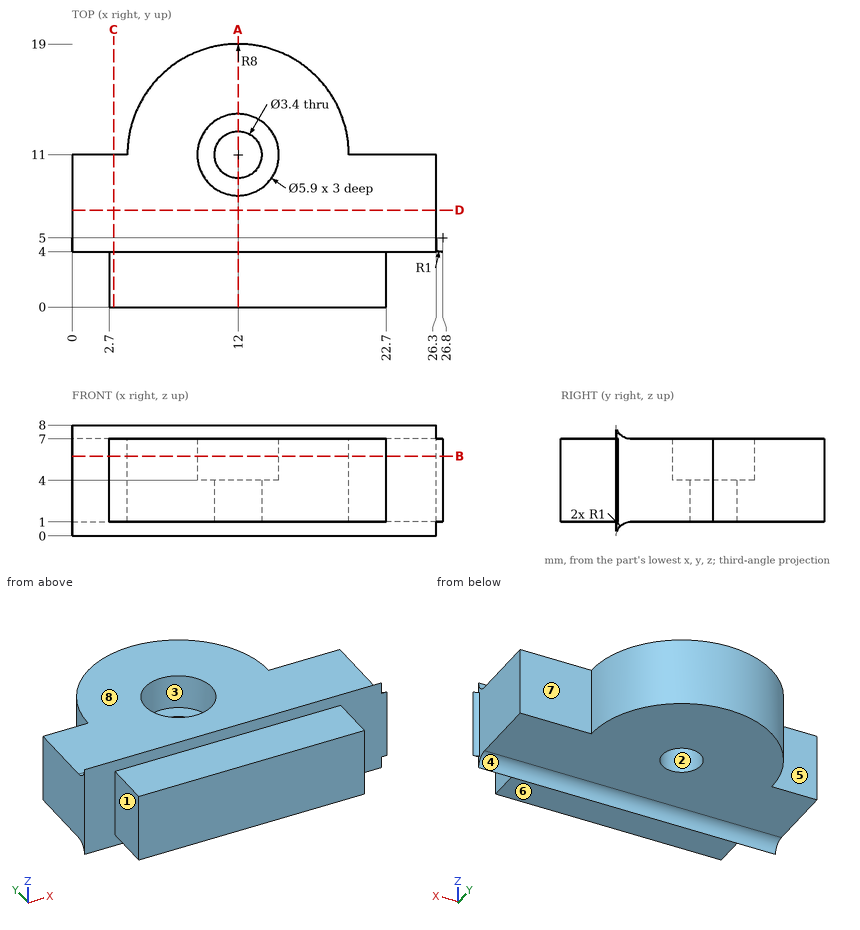
The drawing under review shows one solid part. Ordinate dimensions are in mm from its lowest x, y, z. A direction names the side the tool comes from. Round coordinates to 2 decimals unless told otherwise and drop trailing zeros. Write each loop counter-clockwise with the first axis right and the second up, starting at its lowest first coordinate (ties: lowest second). Pieces come first, ordered by that corner, then holes. Notation, with made-up numbers: (41, 22.25) - (58, 22.25) arc R22 ccw to (58, 35.25) - close; hole circle Ø6 at (54.25, 83). An arc over 180 degrees is marked (long way). Use one line per item in the form item = value.
Q1. Insertion check: pin 1 Ø1.5 at (x, y) = (12.5, 4) entering from -Z; pin 2 Ø2 at (y, z) = (10, 3) entering from +X; pin 3 Ø2 at (x, y) = (14, 2.5) entering from -Z; pin 4 Ø2 at (x, z) = (6, 5.5) entering from -Y. Each pin has a flat end and moves straight along its axis. Give the tip position at first contact, or say it passes through.
Answer key:
pin_1 = 0
pin_2 = 26.3
pin_3 = 1
pin_4 = 0
Q2. Consider section A-A (x = 12). State the section outline as (y, z) points, and give its area (3 significant figures).
Answer key:
outline = (0, 1) - (4, 1) - (4, 0) arc R1 cw to (5, 1) - (9.3, 1) - (9.3, 4) - (8.05, 4) - (8.05, 7) - (5, 7) arc R1 cw to (4, 8) - (4, 7) - (0, 7) - close; (12.7, 1) - (19, 1) - (19, 7) - (13.95, 7) - (13.95, 4) - (12.7, 4) - close
area = 86.5 mm2
Q3. Consider section D-D (y = 7). State the section outline as (x, z) points.
Answer key:
outline = (0, 1) - (26.3, 1) - (26.3, 7) - (0, 7) - close
Q4. Draft analysis for pull direction X (two halves, no side actions). For the marked faces 1, 2, 3 and 4, state which applies: +X half, -X half, draft (parallel to the pull), parting line (faces both ways), or undercut.
Answer key:
face_1 = -X half
face_2 = undercut
face_3 = undercut
face_4 = draft
Q5. Tool access review of the marked faces 5, 6, 7 and 8: name each direction out of +Z, -Z, +X, -X, +Y, -Y from which nothing blocks a thin tool from reaching the whole face with its end or side.
Answer key:
face_5 = +Z, -Z, -X, +Y
face_6 = -Z, +X, -X, -Y
face_7 = +Z, -Z, +X, +Y
face_8 = +Z, +X, -X, +Y
Q6. Consider section C-C (x = 3). State the section outline as (y, z) points, and give its area (3 significant figures).
Answer key:
outline = (0, 1) - (4, 1) - (4, 0) arc R1 cw to (5, 1) - (11, 1) - (11, 7) - (5, 7) arc R1 cw to (4, 8) - (4, 7) - (0, 7) - close
area = 66.4 mm2
Q7. For line 1 (Y direction, x = 12, z = 1.8); line 2 (Z direction, x = 2.25, y = 7.75); line 3 (X direction, y = 7, z = 4.5), list the stretches that pass through material, from the lowest coordinate up. Write a range as [from, to].
Answer key:
line_1 = [0, 9.3], [12.7, 19]
line_2 = [1, 7]
line_3 = [0, 26.3]
Q8. Consider section B-B (z = 5.75). State the section outline as (x, y) points.
Answer key:
outline = (0, 4) - (2.7, 4) - (2.7, 0) - (22.7, 0) - (22.7, 4) - (26.8, 4) arc R1 cw to (26.3, 4.13) - (26.3, 11) - (20, 11) arc R8 ccw to (4, 11) - (0, 11) - close; hole circle Ø5.9 at (12, 11)
